Autodesk Inventor part; units mm, degrees
ref_plane "YZ Plane" through (0, 0, 0) normal (1, 0, 0) x (0, 1, 0)
ref_plane "XZ Plane" through (0, 0, 0) normal (0, 1, 0) x (-1, 0, 0)
ref_plane "XY Plane" through (0, 0, 0) normal (0, 0, 1) x (1, 0, 0)
sketch "Sketch1" plane through (0, 0, 0) normal (0, 0, 1) x (1, 0, 0)
  line L0 (-60, 40) -> (60, 40)
  line L1 (60, 40) -> (60, -40)
  line L2 (60, -40) -> (-60, -40)
  line L3 (-60, -40) -> (-60, 40)
  point P0 (0, 0)
  point P1 (-60, 0)
  point P2 (0, 40)
  dimension "d0" = 120
  dimension "d1" = 80
extrude "Extrusion1" add sketch "Sketch1" along normal blind 80
sketch "Sketch4" plane through (-60, -40, 0) normal (-1, 0, 0) x (0, 0, 1)
  circle A0 centre (40, 40) radius 15
  line L0 (0, 0) -> (0, 80)
  line L1 (0, 80) -> (80, 80)
  point P0 (0, 40)
  point P1 (0, 40)
  point P2 (40, 80)
  dimension "d12" = 30
extrude "Extrusion2" add sketch "Sketch4" along normal blind 35
sketch "Sketch7" plane through (-95, 0, 40) normal (-1, 0, 0) x (0, 0, 1)
  circle A0 centre (0, 0) radius 15
  line L0 (0, 15) -> (15, 0)
  line L1 (0, -15) -> (15, 0)
  line L2 (0, -15) -> (-15, 0)
  line L3 (0, 15) -> (-15, 0)
  point P0 (-40, 0)
extrude "Extrusion3" cut sketch "Sketch7" against normal blind 30 contours L0 A0 | A0 L1 | L3 A0 | A0 L2
sketch "Sketch8" plane through (60, -40, 0) normal (1, 0, 0) x (0, 0, -1)
  line L0 (-50, 25) -> (-30, 25)
  line L1 (-30, 25) -> (-30, 55)
  line L2 (-30, 55) -> (-50, 55)
  line L3 (-50, 55) -> (-50, 25)
  line L4 (0, 0) -> (-80, 0)
  line L5 (-80, 0) -> (-80, 80)
  line L6 (-38, 33) -> (-42, 33)
  line L7 (-42, 33) -> (-42, 28)
  line L8 (-42, 28) -> (-38, 28)
  line L9 (-38, 28) -> (-38, 33)
  line L10 (-37, 40) -> (-43, 40)
  line L11 (-43, 40) -> (-43, 36)
  line L12 (-43, 36) -> (-37, 36)
  line L13 (-37, 36) -> (-37, 40)
  line L14 (-37, 46) -> (-43, 46)
  line L15 (-43, 46) -> (-43, 42)
  line L16 (-43, 42) -> (-37, 42)
  line L17 (-37, 42) -> (-37, 46)
  line L18 (-44, 49) -> (-36, 49)
  line L19 (-36, 49) -> (-36, 52)
  line L20 (-36, 52) -> (-44, 52)
  line L21 (-44, 52) -> (-44, 49)
  point P0 (0, 40)
  point P1 (-40, 25)
  point P2 (-40, 0)
  point P3 (-50, 40)
  point P4 (-80, 40)
  point P5 (-40, 28)
  point P6 (-40, 36)
  point P7 (-40, 42)
  point P8 (-40, 52)
  point P9 (-40, 55)
  dimension "d17" = 30
  dimension "d18" = 20
  dimension "d19" = 5
  dimension "d20" = 4
  dimension "d21" = 4
  dimension "d22" = 6
  dimension "d23" = 6
  dimension "d24" = 4
  dimension "d27" = 3
  dimension "d28" = 8
  dimension "d29" = 3
  dimension "d30" = 2
  dimension "d31" = 3
  dimension "d32" = 3
extrude "Extrusion4" cut sketch "Sketch8" against normal blind 5
sketch "Sketch9" plane through (0, 0, 80) normal (0, 0, 1) x (1, 0, 0)
  circle A0 centre (-55, 35) radius 2.5
  line L0 (-60, 40) -> (-60, -40)
  line L1 (60, 40) -> (-60, 40)
  circle A1 centre (55, 35) radius 2.5
  circle A2 centre (-55, -35) radius 2.5
  circle A3 centre (55, -35) radius 2.5
  point P0 (0, 0)
  dimension "d35" = 5
  dimension "d36" = 5
  dimension "d37" = 5
  dimension "d40" = 110
  dimension "d43" = 70
extrude "Extrusion5" cut sketch "Sketch9" against normal blind 5
properties part number "motor"
Verification items for the finished model (mm, model axes). A direction names the side the tool comes from. Coordinates: 2 decimals unless noted, no trailing zeros. Order: outer loops, then holes, each group sorted by start corner. A loop starts at its lowest first (then second) coordinate and runs counter-clockwise, first axis right, second up. Notation, with made-up numbers: M 65,29.5 L 123,29.5 A5 cw 123,37.5 Z; hole C 64.5,10.25 d3. An arc over 180 degrees is marked long. One line per item, written item: value. Start each with the question number.
Item 1: Sectioned sample at A-A (y = 35). Enter the section's corners in (x, z), then the cut area to 3 significant figures.
Item 2: Sectioned sample at C-C (z = 18). Enter the section's corners in (x, y), then the cut area to 3 significant figures.
Item 3: Access from +Z, -Z, +X, -X, +Y, -Y to the whole of each face (thin tool, end or side, straight path). Record for faces 1 (the cylindrical face through (57.385, -34.249, 77.535)), 2 (the cylindrical face through (-62.465, -0.66, 25.015)), 3 (the flat face through (58, 10, 36)), 4 (the flat face through (-80, 8, 33)).
Item 4: Sectioned sample at B-B (z = 47). Enter the section's corners in (x, y).
Item 5: Scan lines: probe 1 along Y at (x, z) = (55, 76.65); probe 2 along X at (y, z) = (33.5, 30); probe 3 along X at (y, z) = (-3.5, 28). Record each from-to range of solid material in increasing order.
Item 6: Gauge pin test, flat ends, axial feed: pin 1 (1.5 mm diameter, centred on y = 25, z = 70, fed in from -X); pin 2 (2.5 mm diameter, centred on x = 55.5, y = -35, fed in from +Z). Record the tip position at first contact, or that the pin passes through.
Item 7: Mould release check, pull along X, two halves, no side actions. Record for faces 5 (the flat face through (58, 0, 40)), 6 (the flat face through (60, 4, 40)), 7 (the cylindrical face through (57.31, 34.04, 77.54)): released by +X, released by -X, zero draft, split by the parting line, or undercut.
Conclusion:
1. outline: M -60,0 L 60,0 L 60,80 L 57.5,80 L 57.5,75 L 52.5,75 L 52.5,80 L -52.5,80 L -52.5,75 L -57.5,75 L -57.5,80 L -60,80 Z
1. area: 9,550 mm^2
2. outline: M -60,-40 L 60,-40 L 60,40 L -60,40 Z
2. area: 9,600 mm^2
3. face 1: +Z
3. face 2: -X
3. face 3: +X
3. face 4: -Z, -X, +Y
4. outline: M -95,-8 L -65,-8 L -65,-13.27 L -60,-13.27 L -60,-40 L 60,-40 L 60,-15 L 55,-15 L 55,15 L 60,15 L 60,40 L -60,40 L -60,13.27 L -65,13.27 L -65,8 L -95,8 Z
5. probe 1: y = -40 to -37.5, -32.5 to 32.5, 37.5 to 40
5. probe 2: x = -60 to 60
5. probe 3: x = -65 to 60
6. pin 1: stops at x = -60
6. pin 2: stops at z = 75
7. face 5: zero draft
7. face 6: released by +X
7. face 7: undercut
